Source: CAD feature listing. Evaluate the final solid. Frame: model axes, mm. Give positions to 0.01 mm unless a question says otherwise; leave off trailing zeros. Loops run counter-clockwise (first coordinate to the right, second up) from the corner with the lowest first, then second, coordinate; pieces in that order, holes last.
```python
from build123d import *

# Parameters (mm, degrees)
F1_DEPTH = 25.4


with BuildPart() as f1:
    # F0 (on Front) → F1 (new body)
    with BuildSketch(Plane.XZ):
        Polygon((0, 31.75), (-11.556055, 31.75), (-29.260958, 16.893822), (-33.274334, -5.867163), (-21.718279, -25.882837), (0, -33.787644), (21.718279, -25.882837), (33.274334, -5.867163), (29.260958, 16.893822), (11.556055, 31.75), align=None)
    extrude(amount=F1_DEPTH)


solid = f1.part
```
(1) First-contact query: pin 1 (12 mm diameter, centred on y = -4.5, z = 1, fed in from +X); pin 2 (2 mm diameter, centred on x = 25, y = -20.5, fed in from +Z); pin 3 (4 mm diameter, centred on x = -16.5, y = -16, fed in from -Z). Flat tips, straight axial feed; report the tip coordinate or a pass-through.
A:
pin 1: stops at x = 33.12
pin 2: stops at z = 21.31
pin 3: stops at z = -28.51
(2) Section B-B, the plane x = 19. Return the cut outline in (y, z), then the cut area to 3 significant figures.
A:
outline: (-25.4, -26.87) - (0, -26.87) - (0, 25.5) - (-25.4, 25.5) - close
area: 1,330 mm2
(3) Section C-C, the plane z = 23. Return the cut outline in (x, y).
A:
outline: (-21.98, -25.4) - (21.98, -25.4) - (21.98, 0) - (-21.98, 0) - close
(4) Ray query, line 1 along X through (y, z) = (-14, -3); line 2 along Z through (x, y) = (15, -6.5); line 3 along Z through (x, y) = (-2, -4.5). Return the intervals inside material, ascending.
A:
line 1: x = -32.77 to 32.77
line 2: z = -28.33 to 28.86
line 3: z = -33.06 to 31.75
(5) Section A-A, the plane y = -8. Return the cut outline in (x, z).
A:
outline: (-33.27, -5.87) - (-21.72, -25.88) - (0, -33.79) - (21.72, -25.88) - (33.27, -5.87) - (29.26, 16.89) - (11.56, 31.75) - (-11.56, 31.75) - (-29.26, 16.89) - close
